Drawing for the job (mm, zero at the part's lowest x, y, z). Give positions to 0.01 mm unless a question says otherwise; leave off trailing zeros. Loops run counter-clockwise (first coordinate to the right, second up) from the corner with the lowest first, then second, coordinate; pieces in that order, holes last. Notation, with made-up numbers: (-22.75, 78.25) - (-8.75, 78.25) arc R6 cw to (-8.75, 82.25) - close; hole circle Ø5 at (21.5, 54.25). An arc over 180 degrees is marked (long way). Return JSON: item names as keys, results as strings. Group by question number.
1) Slice it at A-A (y = 63.5). List the corners of the cut face in (x, z) (3 decimals), and give its area (3 significant figures).
2) Drill centre line: probe 1 along Y at (x, z) = (127, 12.25) (3 decimals). Where is it in solid material? Low to high. Write a range as from..to.
3) Drop a flat-ended pin along its axis: pin 1 (5 mm diameter, centred on x = 76.2, y = 63.5, fed in from -Z). Give the stop position or say it passes through.
4) Slice it at B-B (x = 177.8). List the corners of the cut face in (y, z) (3 decimals), and give its area (3 significant figures).
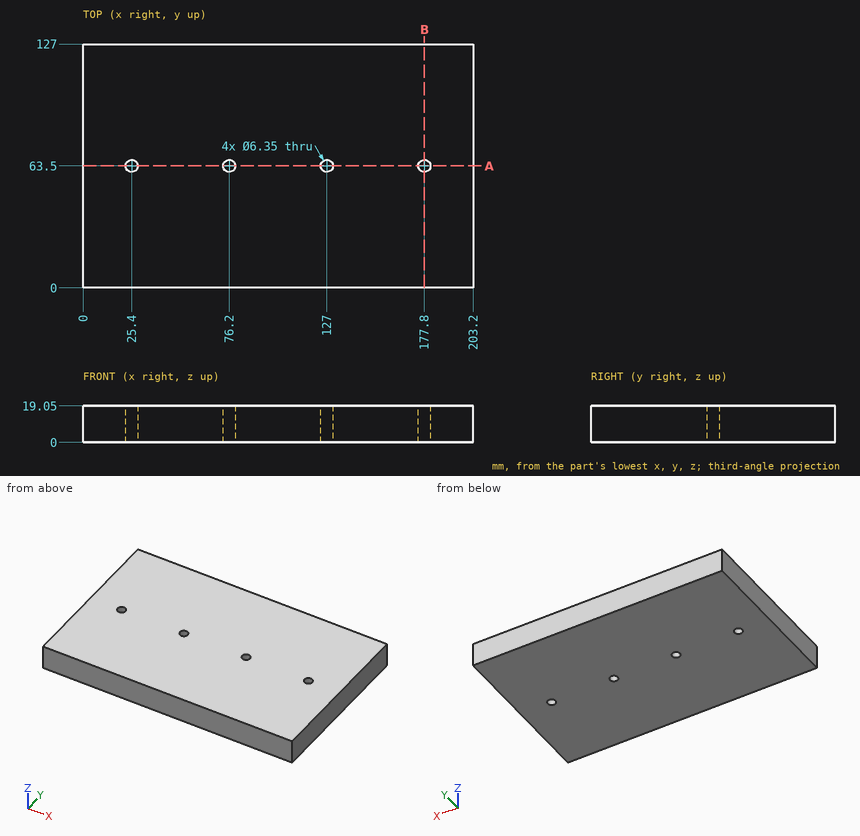
Results:
{
 "1": {"outline": "(0, 0) - (22.225, 0) - (22.225, 19.05) - (0, 19.05) - close; (28.575, 0) - (73.025, 0) - (73.025, 19.05) - (28.575, 19.05) - close; (79.375, 0) - (123.825, 0) - (123.825, 19.05) - (79.375, 19.05) - close; (130.175, 0) - (174.625, 0) - (174.625, 19.05) - (130.175, 19.05) - close; (180.975, 0) - (203.2, 0) - (203.2, 19.05) - (180.975, 19.05) - close", "area": "3,390 mm2"},
 "2": {"probe 1": "0..60.325, 66.675..127"},
 "3": {"pin 1": "through"},
 "4": {"outline": "(0, 0) - (60.325, 0) - (60.325, 19.05) - (0, 19.05) - close; (66.675, 0) - (127, 0) - (127, 19.05) - (66.675, 19.05) - close", "area": "2,300 mm2"}
}
